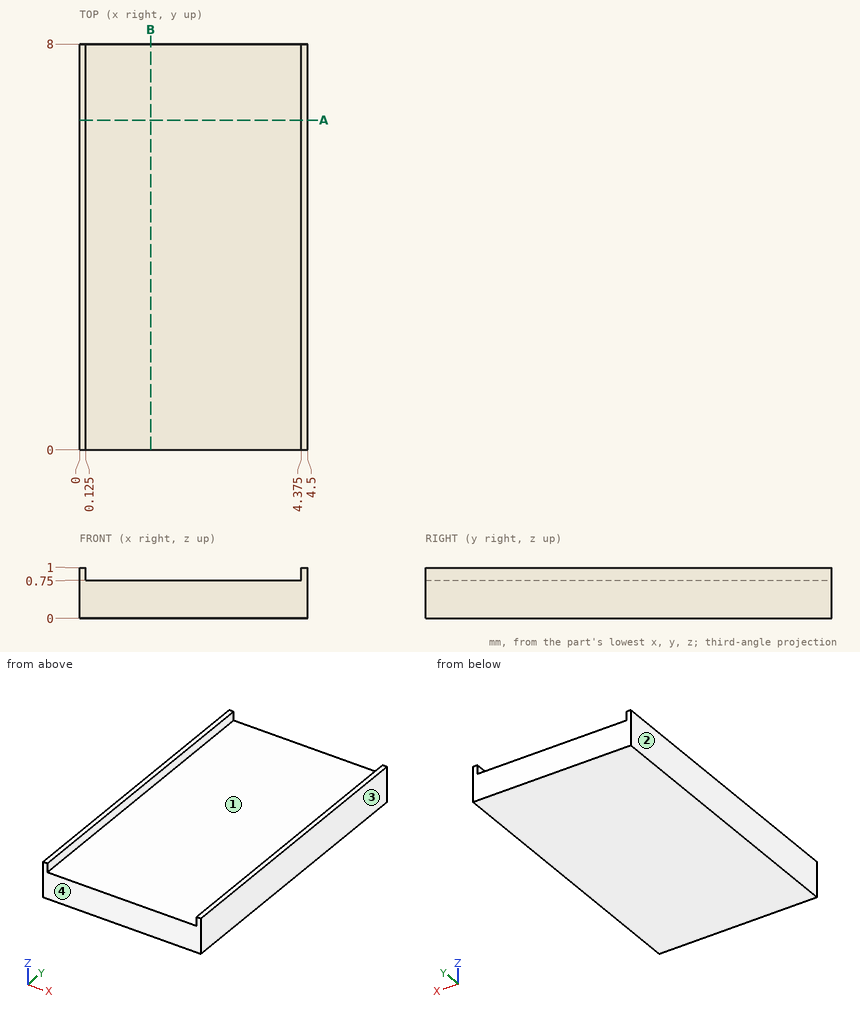
Geometry: see drawing. Coordinates: mm, zero at the bounding-box minimum. Round coordinates to 2 decimals unless told otherwise and drop trailing zeros. Write each loop counter-clockwise with the first axis right and the second up, starting at its lowest first coordinate (ties: lowest second). Pieces come first, ordered by that corner, then holes.
Item 1: Mould query, pull axis X, two halves, no side actions, for the marked faces 1, 2, 3 and 4. Classes: +X half, -X half, draft (parallel to the pull), parting line (faces both ways), or undercut.
Item 2: Section query A-A (y = 6.5). Return loops of the section in (x, z) (3 decimals).
Item 3: Section query B-B (x = 1.4). Return loops of the section in (y, z), plus the area to 3 significant figures.
Item 4: Material intervals for L1, parallel to Z at x = 2.3, y = 1.75, sorted ascending.
Item 5: Pin query (flat end, axial travel): P1, Ø1.3, axis at x = 1.5, y = 5.5, coming from the +Z side. Return the tip coordinate at first contact, or that it passes through.
Completed:
1. face 1: undercut
1. face 2: -X half
1. face 3: +X half
1. face 4: draft
2. outline: (0, 0) - (4.5, 0) - (4.5, 1) - (4.375, 1) - (4.375, 0.75) - (0.125, 0.75) - (0.125, 1) - (0, 1) - close
3. outline: (0, 0) - (8, 0) - (8, 0.75) - (0, 0.75) - close
3. area: 6.00 mm2
4. L1: z = 0 to 0.75
5. P1: stops at z = 0.75
